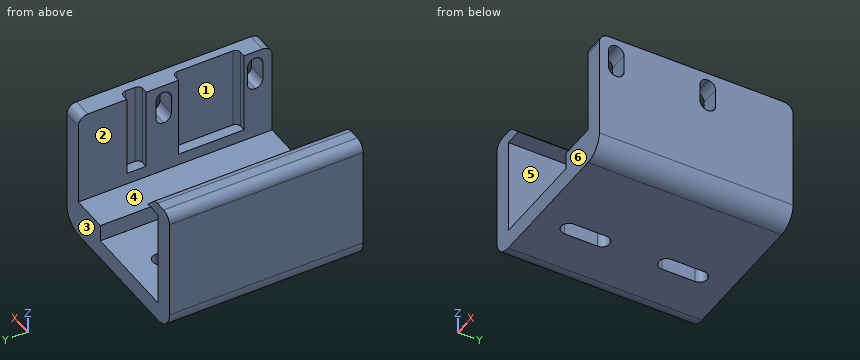
```python
from build123d import *

# Parameters (mm, degrees)
F1_DEPTH  = 40
F2_R      = 4
F3_R      = 2
F4_W      = 3.2
F4_H      = 7
F5_DEPTH  = 4
F6_R      = 1.59999
F7_W      = 3.2
F7_H      = 10
F8_DEPTH  = 4
F9_R      = 1.59999
F10_W     = 2.2
F10_H     = 4
F10_H_2   = 13.5
F11_DEPTH = 17
F12_R     = 2
F13_R     = 1
F14_R     = 2


# Not quite as in the source:
# - a fillet or chamfer is up to 0.001 mm smaller than in the source, because OpenCascade refuses the exact size


with BuildPart() as f1:
    # F0 (on Front) → F1 (new body)
    with BuildSketch(Plane.XZ):
        Polygon((21.0562500745, -30.2744720221), (21.0562500745, -3.3744720221), (17.0562500745, -3.3744720221), (17.0562500745, -22.7744720221), (9.3562500745, -22.7744720221), (9.3562500745, -26.2744720221), (-10.8437499255, -26.2744720221), (-10.8437499255, -6.0744720221), (-7.3437499255, -6.0744720221), (-9.8437499255, -3.5744720221), (-14.8437499255, -3.5744720221), (-14.8437499255, -30.2744720221), align=None)
    extrude(amount=F1_DEPTH)

    # F2
    f2_edges = [f1.edges().sort_by_distance(p)[0] for p in [
        (-14.84375, -20, -30.274472),
        (21.05625, -20, -30.274472),
    ]]
    fillet(f2_edges, radius=F2_R)

    # F3
    f3_edges = [f1.edges().sort_by_distance(p)[0] for p in [
        (-9.84375, -20, -3.574472),
    ]]
    fillet(f3_edges, radius=F3_R)

    # F4 (on face) → F5 (cut, through all)
    with BuildSketch(Plane.YZ.offset(21.0562500745)):
        with Locations((-17.6, -8.3744720221)):
            Rectangle(F4_W, F4_H)
        with Locations((-36.5, -8.3744720221)):
            Rectangle(F4_W, F4_H)
    extrude(amount=-F5_DEPTH, mode=Mode.SUBTRACT)

    # F6 (radius 1.6 in the source; OpenCascade refuses exactly that, so slightly less here)
    f6_edges = [f1.edges().sort_by_distance(p)[0] for p in [
        (19.05625, -19.2, -4.874472),
        (19.05625, -16, -4.874472),
        (19.05625, -16, -11.874472),
        (19.05625, -19.2, -11.874472),
        (19.05625, -38.1, -11.874472),
        (19.05625, -34.9, -11.874472),
        (19.05625, -34.9, -4.874472),
        (19.05625, -38.1, -4.874472),
    ]]
    fillet(f6_edges, radius=F6_R)

    # F7 (on face) → F8 (cut, through all)
    with BuildSketch(Plane(origin=(0, 0, -30.2744720221), x_dir=(1, 0, 0), z_dir=(0, 0, -1))):
        with Locations((-0.500000006, 10)):
            Rectangle(F7_W, F7_H)
        with Locations((-0.7437499255, 30)):
            Rectangle(F7_W, F7_H)
    extrude(amount=-F8_DEPTH, mode=Mode.SUBTRACT)

    # F9 (radius 1.6 in the source; OpenCascade refuses exactly that, so slightly less here)
    f9_edges = [f1.edges().sort_by_distance(p)[0] for p in [
        (0.85625, -35, -28.274472),
        (-2.34375, -35, -28.274472),
        (-2.1, -15, -28.274472),
        (1.1, -15, -28.274472),
        (0.85625, -25, -28.274472),
        (1.1, -5, -28.274472),
        (-2.34375, -25, -28.274472),
        (-2.1, -5, -28.274472),
    ]]
    fillet(f9_edges, radius=F9_R)

    # F10 (on face) → F11 (cut)
    with BuildSketch(Plane.XY.offset(-3.3744720221)):
        with Locations((18.1562500745, -12)):
            Rectangle(F10_W, F10_H)
        with Locations((18.1562500745, -27.45)):
            Rectangle(F10_W, F10_H_2)
    extrude(amount=-F11_DEPTH, mode=Mode.SUBTRACT)

    # F12
    f12_edges = [f1.edges().sort_by_distance(p)[0] for p in [
        (19.05625, -40, -3.374472),
        (19.05625, 0, -3.374472),
    ]]
    fillet(f12_edges, radius=F12_R)

    # F13
    f13_edges = [f1.edges().sort_by_distance(p)[0] for p in [
        (19.25625, -14, -11.874472),
        (19.25625, -10, -11.874472),
        (19.25625, -20.7, -11.874472),
        (19.25625, -34.2, -11.874472),
    ]]
    fillet(f13_edges, radius=F13_R)

    # F14
    f14_edges = [f1.edges().sort_by_distance(p)[0] for p in [
        (-14.84375, -20, -3.574472),
    ]]
    fillet(f14_edges, radius=F14_R)


solid = f1.part
```
For this review, take the finished solid that the model builds, in its own axes (mm). Face numbers are marked on the shaded views. A direction names the side the tool comes from. Coordinates: 2 decimals unless noted, no trailing zeros. Order: outer loops, then holes, each group sorted by start corner. A loop starts at its lowest first (then second) coordinate and runs counter-clockwise, first axis right, second up. Notation, with made-up numbers: (53.25, 68) -> (85.25, 68) arc R22 ccw to (85.25, 91) -> close; hole circle Ø5 at (-33, 42). An arc over 180 degrees is marked (long way). Use CSV: the item, a comma, the result in double quotes. Start each with the question number.
Item 1: We need section B-B, the plane y = -7.5. Give the boundary of the cut face in (x, z), then the cut area to 3 significant figures.
Item 2: We need section A-A, the plane z = -17. Give the boundary of the cut face in (x, y), then the cut area to 3 significant figures.
Item 3: We need section C-C, the plane x = -8. Give the boundary of the cut face in (y, z).
Item 4: Insertion check: pin 1 (1.8 mm diameter, centred on x = 18, y = -13, fed in from +Z); pin 2 (2 mm diameter, centred on y = -28.5, z = -29, fed in from -X); pin 3 (12 mm diameter, centred on x = 5, y = -27.5, fed in from +Z). Each pin has a flat end and moves straight along its axis. Give the tip position at first contact, or say it passes through.
Item 5: Draft analysis for pull direction Z (two halves, no side actions). For the marked faces 4, 5 and 6, state which applies: pulls with the +Z half, pulls with the -Z half, needs draft (parallel to the pull), parting line crosses it, or undercut.
Item 6: Wall thickness on probe 1 along X at (y, z) = (-5, -25.25); probe 2 along X at (y, z) = (-15, -20.25); probe 3 along Z at (x, y) = (-7.5, -17): over which ranges is each line inside the solid? List them lowest first.
Item 7: For the marked faces 1, 2 and 3, list the 3-axis set-ups (+Z, -Z, +X, -X, +Y, -Y) from which the entire face can be reached by the end or side of a thin tool; tool diameter is ignored.
Item 8: We need section D-D, the plane y = -30. Give the boundary of the cut face in (x, z).
Derived:
1,outline,"(-14.84, -26.27) arc R4 ccw to (-10.84, -30.27) -> (-2.1, -30.27) -> (-2.1, -26.27) -> (-10.84, -26.27) -> (-10.84, -6.07) -> (-7.34, -6.07) -> (-9.26, -4.16) arc R2 ccw to (-10.67, -3.57) -> (-12.84, -3.57) arc R2 ccw to (-14.84, -5.57) -> close; (1.1, -30.27) -> (17.06, -30.27) arc R4 ccw to (21.06, -26.27) -> (21.06, -3.37) -> (17.06, -3.37) -> (17.06, -22.77) -> (9.36, -22.77) -> (9.36, -26.27) -> (1.1, -26.27) -> close"
1,area,"338 mm^2"
2,outline,"(-14.84, -40) -> (-10.84, -40) -> (-10.84, 0) -> (-14.84, 0) -> close; (17.06, -40) -> (21.06, -40) -> (21.06, 0) -> (17.06, 0) -> (17.06, -10) -> (18.26, -10) arc R1 cw to (19.26, -11) -> (19.26, -13) arc R1 cw to (18.26, -14) -> (17.06, -14) -> (17.06, -20.7) -> (18.26, -20.7) arc R1 cw to (19.26, -21.7) -> (19.26, -33.2) arc R1 cw to (18.26, -34.2) -> (17.06, -34.2) -> close"
2,area,"282 mm^2"
3,outline,"(-40, -30.27) -> (0, -30.27) -> (0, -26.27) -> (-40, -26.27) -> close; (-40, -6.07) -> (0, -6.07) -> (0, -5.42) -> (-40, -5.42) -> close"
4,pin 1,"stops at z = -20.37"
4,pin 2,"stops at x = -14.45"
4,pin 3,"stops at z = -22.77"
5,face 4,"pulls with the +Z half"
5,face 5,"undercut"
5,face 6,"needs draft"
6,probe 1,"x = -14.84 to -10.84, 9.36 to 21.06"
6,probe 2,"x = -14.84 to -10.84, 17.06 to 21.06"
6,probe 3,"z = -30.27 to -26.27, -6.07 to -5.92"
7,face 1,"+Z"
7,face 2,"+Z, +Y, -Y"
7,face 3,"+Z, -Z, +X, -X, +Y"
8,outline,"(-14.84, -26.27) arc R4 ccw to (-10.84, -30.27) -> (-2.34, -30.27) -> (-2.34, -26.27) -> (-10.84, -26.27) -> (-10.84, -6.07) -> (-7.34, -6.07) -> (-9.26, -4.16) arc R2 ccw to (-10.67, -3.57) -> (-12.84, -3.57) arc R2 ccw to (-14.84, -5.57) -> close; (0.86, -30.27) -> (17.06, -30.27) arc R4 ccw to (21.06, -26.27) -> (21.06, -3.37) -> (19.26, -3.37) -> (19.26, -20.37) -> (17.06, -20.37) -> (17.06, -22.77) -> (9.36, -22.77) -> (9.36, -26.27) -> (0.86, -26.27) -> close"
